from build123d import *

# Parameters (mm, degrees)
SZKIC1_W                    = 21
SZKIC1_H                    = 6
SZKIC1_H_2                  = 20
SZKIC1_R                    = 2.7
DODANIE_WYCI_GNI_CIE1_DEPTH = 6
SZKIC2_W                    = 21
SZKIC2_H                    = 6
DODANIE_WYCI_GNI_CIE2_DEPTH = 20
SZKIC3_R                    = 2.7
WYTNIJ_WYCI_GNI_CIE1_DEPTH  = 9
SZKIC4_W                    = 15
SZKIC4_H                    = 6
DODANIE_WYCI_GNI_CIE3_DEPTH = 22
SZKIC8_R                    = 4.5
SZKIC8_R_2                  = 2.7
DODANIE_WYCI_GNI_CIE6_DEPTH = 3.7
SZKIC9_W                    = 6
SZKIC9_H                    = 18.65
DODANIE_WYCI_GNI_CIE7_DEPTH = 17
ZAOKR_GLENIE3_R             = 6
WYTNIJ_WYCI_GNI_CIE2_DEPTH  = 22
ZAOKR_GLENIE4_R             = 6
SZKIC6_R                    = 4.5
SZKIC6_R_2                  = 2.7
DODANIE_WYCI_GNI_CIE5_DEPTH = 3.7


with BuildPart() as part:
    # Szkic1 → Dodanie-wyciągnięcie1 (new body)
    with BuildSketch(Plane.XY):
        with Locations((10.5, 23)):
            Rectangle(SZKIC1_W, SZKIC1_H)
        with Locations((10.5, 10)):
            Rectangle(SZKIC1_W, SZKIC1_H_2)
        with Locations((13, 10)):
            Circle(SZKIC1_R, mode=Mode.SUBTRACT)
    extrude(amount=DODANIE_WYCI_GNI_CIE1_DEPTH)

    # Szkic2 → Dodanie-wyciągnięcie2 (add)
    with BuildSketch(Plane(origin=(0, 0, 0), x_dir=(-1, 0, 0), z_dir=(0, 0, -1))):
        with Locations((-10.5, 23)):
            Rectangle(SZKIC2_W, SZKIC2_H)
    extrude(amount=DODANIE_WYCI_GNI_CIE2_DEPTH)

    # Szkic3 → Wytnij-wyciągnięcie1 (cut)
    with BuildSketch(Plane(origin=(0, 26, 0), x_dir=(1, 0, 0), z_dir=(0, 1, 0))):
        with Locations((10.5, 10)):
            Circle(SZKIC3_R)
    extrude(amount=-WYTNIJ_WYCI_GNI_CIE1_DEPTH, mode=Mode.SUBTRACT)

    # Szkic4 → Dodanie-wyciągnięcie3 (add)
    with BuildSketch(Plane.XY.offset(6)):
        with Locations((7.5, 21.65)):
            Rectangle(SZKIC4_W, SZKIC4_H)
    extrude(amount=DODANIE_WYCI_GNI_CIE3_DEPTH)

    # Szkic8 → Dodanie-wyciągnięcie6 (add)
    with BuildSketch(Plane(origin=(0, 26, 0), x_dir=(1, 0, 0), z_dir=(0, 1, 0))):
        with Locations((10.5, 10)):
            Circle(SZKIC8_R)
        with Locations((10.5, 10)):
            Circle(SZKIC8_R_2, mode=Mode.SUBTRACT)
    extrude(amount=DODANIE_WYCI_GNI_CIE6_DEPTH)

    # Szkic9 → Dodanie-wyciągnięcie7 (add)
    with BuildSketch(Plane.XY.offset(6)):
        with Locations((3, 9.325)):
            Rectangle(SZKIC9_W, SZKIC9_H)
    extrude(amount=DODANIE_WYCI_GNI_CIE7_DEPTH)

    # Zaokrąglenie3
    zaokr_glenie3_edges = [part.edges().sort_by_distance(p)[0] for p in [
        (3, 0, 23),
    ]]
    fillet(zaokr_glenie3_edges, radius=ZAOKR_GLENIE3_R)

    # Szkic12 → Wytnij-wyciągnięcie2 (cut)
    with BuildSketch(Plane(origin=(0, 24.65, 0), x_dir=(1, 0, 0), z_dir=(0, 1, 0))):
        with BuildLine():
            Line((12, -14.55), (7.5, -14.55))
            ThreePointArc((7.5, -14.55), (6.25, -13.3), (7.5, -12.05))
            Line((7.5, -12.05), (12, -12.05))
            ThreePointArc((12, -12.05), (13.25, -13.3), (12, -14.55))
        make_face()
        with BuildLine():
            Line((12, -21.45), (7.5, -21.45))
            ThreePointArc((7.5, -21.45), (6.25, -22.7), (7.5, -23.95))
            Line((7.5, -23.95), (12, -23.95))
            ThreePointArc((12, -23.95), (13.25, -22.7), (12, -21.45))
        make_face()
    extrude(amount=-WYTNIJ_WYCI_GNI_CIE2_DEPTH, mode=Mode.SUBTRACT)

    # Zaokrąglenie4
    zaokr_glenie4_edges = [part.edges().sort_by_distance(p)[0] for p in [
        (21, 23, -20),
    ]]
    fillet(zaokr_glenie4_edges, radius=ZAOKR_GLENIE4_R)

    # Szkic6 → Dodanie-wyciągnięcie5 (add)
    with BuildSketch(Plane(origin=(0, 26, 0), x_dir=(1, 0, 0), z_dir=(0, 1, 0))):
        with Locations((10.5, 10)):
            Circle(SZKIC6_R)
        with Locations((10.5, 10)):
            Circle(SZKIC6_R_2, mode=Mode.SUBTRACT)
    extrude(amount=DODANIE_WYCI_GNI_CIE5_DEPTH)


solid = part.part
Part model, mm, in its own coordinate system. A direction names the side the tool comes from. Coordinates: 2 decimals unless noted, no trailing zeros. Order: outer loops, then holes, each group sorted by start corner. A loop starts at its lowest first (then second) coordinate and runs counter-clockwise, first axis right, second up.
(1) Slice it at C-C, the plane z = 7. Write the cut outline in (x, y).
Check sheet entries:
outline: (0, 0) - (6, 0) - (6, 18.65) - (15, 18.65) - (15, 24.65) - (0, 24.65) - close
(2) Probe L1, parallel to Z at x = 10.5, y = 22.8; L2, parallel to X at y = 21.85, z = -10; L3, parallel to Y at x = 13, z = 2.8. List the from-to ranges inside material, lowest first.
Check sheet entries:
L1: z = -20 to -12.7, -7.3 to 12.05, 14.55 to 21.45, 23.95 to 28
L2: x = 0 to 7.8, 13.2 to 21
L3: y = 0 to 7.3, 12.7 to 26
(3) Pull direction Z, two halves, no side cores. Call faces 5 (the face through (0, 16, 9)), 6 (the face through (10, 22, 12.05)), 7 (the face through (3, 12, 23)): pulls with the +Z half, pulls with the -Z half, needs draft (parallel to the pull), parting line crosses it, or undercut.
Check sheet entries:
face 5: needs draft
face 6: undercut
face 7: pulls with the +Z half
(4) Slice it at D-D, the plane z = -8.5. Write the cut outline in (x, y) (3 decimals), and give its area (3 significant figures).
Check sheet entries:
outline: (0, 20) - (8.255, 20) - (8.255, 29.7) - (6.257, 29.7) - (6.257, 26) - (0, 26) - close; (12.745, 20) - (21, 20) - (21, 26) - (14.743, 26) - (14.743, 29.7) - (12.745, 29.7) - close
area: 114 mm2
(5) Pin check, flat tips, straight feed: pin 1 Ø12 at (x, z) = (9.5, 14.5) entering from +Y; pin 2 Ø6 at (x, y) = (5, 15.5) entering from +Z; pin 3 Ø1 at (x, y) = (17.5, 6.5) entering from +Z. Stop position of each tip, or through.
Check sheet entries:
pin 1: stops at y = 24.65
pin 2: stops at z = 23
pin 3: stops at z = 6
(6) Slice it at B-B, the plane x = 9.25. Write the cut outline in (y, z).
Check sheet entries:
outline: (0, 0) - (20, 0) - (20, -7.61) - (29.7, -7.61) - (29.7, -5.68) - (26, -5.68) - (26, 6) - (24.65, 6) - (24.65, 12.05) - (18.65, 12.05) - (18.65, 6) - (0, 6) - close; (18.65, 14.55) - (24.65, 14.55) - (24.65, 21.45) - (18.65, 21.45) - close; (18.65, 23.95) - (24.65, 23.95) - (24.65, 28) - (18.65, 28) - close; (20, -20) - (26, -20) - (26, -14.32) - (29.7, -14.32) - (29.7, -12.39) - (20, -12.39) - close
(7) Slice it at A-A, the plane y = 10. Write the cut outline in (x, z), and give its area (3 significant figures).
Check sheet entries:
outline: (0, 0) - (10.3, 0) - (10.3, 6) - (6, 6) - (6, 23) - (0, 23) - close; (15.7, 0) - (21, 0) - (21, 6) - (15.7, 6) - close
area: 196 mm2
(8) Tool access for faces 1 (the face through (13, 13, 6)), 2 (the face through (10, 22, 23.95)), 3 (the face through (8, 20, -8)), 4 (the face through (15, 22, 17)): list every direction of +Z, -Z, +X, -X, +Y, -Y with a clear straight run to the whole face (end or side of a thin tool).
Check sheet entries:
face 1: +Z, +X
face 2: +Y, -Y
face 3: -Z, +X, -X, -Y
face 4: +Z, +X, +Y, -Y
